Can you work these out from the model? Positions are in its coordinate system, mm. A direction names the side the tool comes from. Coordinates: 2 decimals unless noted, no trailing zeros. Loops run counter-clockwise (first coordinate to the right, second up) from the corner with the lowest first, then second, coordinate; pieces in that order, holes last. Notation, with made-up numbers: (25.25, 0.5) -> (39.25, 0.5) arc R26 ccw to (39.25, 21.5) -> close; hole circle Ø8 at (-3, -26). An arc over 180 degrees is marked (long way). Use one line per item in the form item = value. Start each with the question number.
(1) Imagine slicing it at D-D (x = 22). List the corners of the cut face in (y, z) for me, plus the area to 3 significant figures.
(2) I need wall thicknesses on line 1 (X direction, y = 14.5, z = 4.5) (3 decimals); line 2 (Y direction, x = 1.75, z = 6); line 3 (X direction, y = 11.5, z = 9.5) (3 decimals). Which ranges of each line are inside material? Lowest first, please. Write a range as [from, to].
(3) Imagine slicing it at A-A (z = 8.75). List the corners of the cut face in (x, y) for me (3 decimals).
(4) Thinking about a two-plate mould opening in Y: for faces 6 (the flat face through (23, 12.8, 9)), 7 (the flat face through (5.5, 9.8, 10)), 8 (the flat face through (12, 3.65, 6)), which applies, released by +Y, released by -Y, zero draft, split by the parting line, or undercut?
(5) On a 3-axis mill with a long thin cutter (end or side, diameter ignored), from which of +Z, -Z, +X, -X, +Y, -Y can I reach the whole of each face in a straight line? I mean faces 1 (the flat face through (9, 13, 3)), 2 (the flat face through (26.525, 11, 6)), 3 (the flat face through (18, 6.7, 9)), 4 (the flat face through (7, 5.7, 6)), 5 (the flat face through (23, 10, 10)). Say none if no direction works.
(6) Imagine slicing it at C-C (z = 7.25). List the corners of the cut face in (x, y) for me (3 decimals).
(7) I'm going to push flat-ended pins straight in: pin 1 (2 mm diameter, centred on x = 20, y = 18, fed in from +Z); pin 2 (2.5 mm diameter, centred on x = 5.5, z = 4.5, fed in from +Y); pin 3 (1.4 mm diameter, centred on x = 6, z = 9, fed in from +Y). Where does each tip first touch, or does it pass through?
(8) Imagine slicing it at B-B (y = 9.75). List the corners of the cut face in (x, z) for me (3 decimals), plus the area to 3 significant figures.
```python
from build123d import *

# Parameters (mm, degrees)
PAD004_DEPTH    = 8.2
SKETCH014_W     = 28.5
SKETCH014_H     = 6.1
PAD005_DEPTH    = 1.8
SKETCH015_R     = 2.9
POCKET004_DEPTH = 0.6
SKETCH016_W     = 2.05
SKETCH016_H     = 6.1
POCKET005_DEPTH = 1.8
POCKET006_DEPTH = 4
SKETCH019_R     = 2.55
POCKET008_DEPTH = 7.5
SKETCH020_R     = 7
POCKET_DEPTH    = 3


with BuildPart() as part:
    # Sketch013 → Pad004 (new body)
    with BuildSketch(Plane.XY):
        with BuildLine():
            Line((0, 0), (28.5, 0))
            Line((28.5, 0), (28.5, 22.75))
            Line((28.5, 22.75), (14, 22.75))
            Line((14, 22.75), (14, 22.5))
            ThreePointArc((11, 19.5), (13.12132, 20.37868), (14, 22.5))
            Line((11, 19.5), (0, 19.5))
            Line((0, 19.5), (0, 0))
        make_face()
    extrude(amount=PAD004_DEPTH)

    # Sketch014 (on Face9 of Pad004) → Pad005 (join)
    with BuildSketch(Plane.XY.offset(8.2)):
        with Locations((14.25, 9.75)):
            Rectangle(SKETCH014_W, SKETCH014_H)
    extrude(amount=PAD005_DEPTH)

    # Sketch015 (on Face11 of Pad005) → Pocket004 (cut)
    with BuildSketch(Plane.XY.offset(10)):
        with Locations((8.735056, 9.75)):
            Circle(SKETCH015_R)
    extrude(amount=-POCKET004_DEPTH, mode=Mode.SUBTRACT)

    # Sketch016 (on Face10 of Pocket004) → Pocket005 (cut)
    with BuildSketch(Plane.XY.offset(10)):
        with Locations((15.5, 9.75)):
            Rectangle(SKETCH016_W, SKETCH016_H)
        Polygon((21.525, 12.8), (21.525, 6.7), (19.475, 6.7), (19.475, 12.8), (20.5, 12.8), align=None)
        with Locations((25.5, 9.75)):
            Rectangle(SKETCH016_W, SKETCH016_H)
    extrude(amount=-POCKET005_DEPTH, mode=Mode.SUBTRACT)

    # Sketch017 (on Face19 of Clone) → Pocket006 (cut)
    with BuildSketch(Plane.XY.offset(8.2)):
        with BuildLine():
            Line((0, 5.7), (13.475, 5.7))
            ThreePointArc((13.475, 5.7), (14.182107, 5.992893), (14.475, 6.7))
            Line((14.475, 6.7), (14.475, 16.75))
            Line((14.475, 16.75), (16.525, 16.75))
            Line((16.525, 16.75), (16.525, 5.7))
            Line((16.525, 5.7), (18.475, 5.7))
            ThreePointArc((18.475, 5.7), (19.182107, 5.992893), (19.475, 6.7))
            Line((19.475, 6.7), (19.475, 16.75))
            Line((19.475, 16.75), (21.525, 16.75))
            Line((21.525, 16.75), (21.525, 5.699968))
            Line((21.525, 5.699968), (23.475, 5.699968))
            ThreePointArc((23.475, 5.699968), (24.182107, 5.992862), (24.475, 6.699968))
            Line((24.475, 6.699968), (24.475, 16.75))
            Line((24.475, 16.75), (26.525, 16.75))
            Line((26.525, 16.75), (26.525, 5.7))
            ThreePointArc((24.475, 3.65), (25.924569, 4.250431), (26.525, 5.7))
            Line((24.475, 3.65), (0, 3.65))
            Line((0, 3.65), (0, 5.7))
        make_face()
    extrude(amount=-POCKET006_DEPTH, mode=Mode.SUBTRACT)

    # Sketch019 (on Face37 of Pocket006) → Pocket008 (cut)
    with BuildSketch(Plane.XY.offset(9.4)):
        with Locations((8.735056, 9.75)):
            Circle(SKETCH019_R)
    extrude(amount=-POCKET008_DEPTH, mode=Mode.SUBTRACT)

    # Sketch020 (on Face4 of Pocket008) → Pocket (cut)
    with BuildSketch(Plane(origin=(0, 0, 0), x_dir=(1, 0, 0), z_dir=(0, 0, -1))):
        with Locations((8.735056, -9.75)):
            Circle(SKETCH020_R)
    extrude(amount=-POCKET_DEPTH, mode=Mode.SUBTRACT)


solid = part.part
```
Worked out:
q1.outline = (0, 0) -> (22.75, 0) -> (22.75, 8.2) -> (12.8, 8.2) -> (12.8, 10) -> (6.7, 10) -> (6.7, 8.2) -> (5.7, 8.2) -> (5.7, 4.2) -> (3.65, 4.2) -> (3.65, 8.2) -> (0, 8.2) -> close
q1.area = 189 mm2
q2.line_1 = [0, 14.475], [16.525, 19.475], [21.525, 24.475], [26.525, 28.5]
q2.line_2 = [0, 3.65], [5.7, 19.5]
q2.line_3 = [0, 6.423], [11.048, 14.475], [16.525, 19.475], [21.525, 24.475], [26.525, 28.5]
q3.outline = (0, 6.7) -> (14.475, 6.7) -> (14.475, 12.8) -> (0, 12.8) -> close; (16.525, 6.7) -> (19.475, 6.7) -> (19.475, 12.8) -> (16.525, 12.8) -> close; (21.525, 6.7) -> (24.475, 6.7) -> (24.475, 12.8) -> (21.525, 12.8) -> close; (26.525, 6.7) -> (28.5, 6.7) -> (28.5, 12.8) -> (26.525, 12.8) -> close; hole circle Ø5.1 at (8.735, 9.75)
q4.face_6 = released by +Y
q4.face_7 = zero draft
q4.face_8 = undercut
q5.face_1 = -Z
q5.face_2 = +Z
q5.face_3 = +Z, +X, -X, -Y
q5.face_4 = +Z, -X
q5.face_5 = +Z, +X, -X, +Y, -Y
q6.outline = (0, 0) -> (28.5, 0) -> (28.5, 22.75) -> (14, 22.75) -> (14, 22.5) arc R3 cw to (11, 19.5) -> (0, 19.5) -> (0, 5.7) -> (13.475, 5.7) arc R1 ccw to (14.475, 6.7) -> (14.475, 16.75) -> (16.525, 16.75) -> (16.525, 5.7) -> (18.475, 5.7) arc R1 ccw to (19.475, 6.7) -> (19.475, 16.75) -> (21.525, 16.75) -> (21.525, 5.7) -> (23.475, 5.7) arc R1 ccw to (24.475, 6.7) -> (24.475, 16.75) -> (26.525, 16.75) -> (26.525, 5.7) arc R2.05 cw to (24.475, 3.65) -> (0, 3.65) -> close; hole circle Ø5.1 at (8.735, 9.75)
q7.pin_1 = 8.2
q7.pin_2 = 19.5
q7.pin_3 = 12.8
q8.outline = (0, 0) -> (1.735, 0) -> (1.735, 3) -> (6.185, 3) -> (6.185, 9.4) -> (5.835, 9.4) -> (5.835, 10) -> (0, 10) -> close; (11.285, 3) -> (15.735, 3) -> (15.735, 0) -> (28.5, 0) -> (28.5, 10) -> (26.525, 10) -> (26.525, 4.2) -> (24.475, 4.2) -> (24.475, 10) -> (21.525, 10) -> (21.525, 4.2) -> (19.475, 4.2) -> (19.475, 10) -> (16.525, 10) -> (16.525, 4.2) -> (14.475, 4.2) -> (14.475, 10) -> (11.635, 10) -> (11.635, 9.4) -> (11.285, 9.4) -> close
q8.area = 171 mm2
